Source: CAD feature listing. Evaluate the final solid. Frame: model axes, mm. A direction names the side the tool comes from. Give positions to 0.01 mm unless a question says otherwise; leave off trailing zeros. Loops run counter-clockwise (first coordinate to the right, second up) from the corner with the lowest first, then second, coordinate; pieces in that order, holes last. Notation, with made-up numbers: (3.5, 11.25) -> (44.5, 11.25) arc R26 ccw to (44.5, 35.25) -> close; hole circle Ø8 at (-8.75, 76). An arc over 180 degrees is marked (long way). Put each result on its own line as item: value.
```python
from build123d import *

# Parameters (mm, degrees)
SALIENTE_EXTRUIR2_DEPTH    = 25
CROQUIS4_W                 = 40
CROQUIS4_H                 = 40
CORTAR_EXTRUIR1_DEPTH      = 20
CROQUIS5_R                 = 7
CORTAR_EXTRUIR2_DEPTH      = 42
CORTAR_EXTRUIR2_DEPTH_BACK = 2
CROQUIS6_R                 = 4.5
CORTAR_EXTRUIR3_DEPTH      = 51
CORTAR_EXTRUIR3_DEPTH_BACK = 11
CORTAR_EXTRUIR4_DEPTH      = 26
CROQUIS9_R                 = 1.5
CROQUIS9_R_2               = 3
CORTAR_EXTRUIR6_DEPTH      = 61
CROQUIS10_R                = 1.5
CROQUIS10_R_2              = 3
CORTAR_EXTRUIR7_DEPTH      = 52
CORTAR_EXTRUIR7_DEPTH_BACK = 2
CROQUIS11_W                = 17.982621029
CROQUIS11_H                = 22.653478674
CORTAR_EXTRUIR8_DEPTH      = 52
CORTAR_EXTRUIR8_DEPTH_BACK = 2
CROQUIS13_R                = 1
CORTAR_EXTRUIR9_DEPTH      = 70
CROQUIS14_R                = 1
CORTAR_EXTRUIR10_DEPTH     = 70
CROQUIS15_R                = 2
CORTAR_EXTRUIR11_DEPTH     = 1.5
CROQUIS16_R                = 2
CORTAR_EXTRUIR12_DEPTH     = 1.5
CROQUIS18_W                = 2.75
CROQUIS18_H                = 7
CORTAR_EXTRUIR13_DEPTH     = 14


with BuildPart() as part:
    # Croquis3 → Saliente-Extruir2 (new body)
    with BuildSketch(Plane.XY):
        Polygon((-5, 45), (91.5, 50), (120, 50), (120, 45), (91.5, 45), (91.5, -5), (120, -5), (120, -10), (91.5, -10), (-5, -5), align=None)
    extrude(amount=SALIENTE_EXTRUIR2_DEPTH)

    # Croquis4 → Cortar-Extruir1 (cut)
    with BuildSketch(Plane.XY.offset(25)):
        with Locations((20, 20)):
            Rectangle(CROQUIS4_W, CROQUIS4_H)
    extrude(amount=-CORTAR_EXTRUIR1_DEPTH, mode=Mode.SUBTRACT)

    # Croquis5 → Cortar-Extruir2 (cut, two sides)
    with BuildSketch(Plane.XZ.offset(-40)) as cortar_extruir2_sk:
        with BuildLine():
            ThreePointArc((3, 15), (10, 22), (17, 15))
            Line((17, 15), (17, 25))
            Line((17, 25), (3, 25))
            Line((3, 25), (3, 15))
        make_face()
        with Locations((10, 15)):
            Circle(CROQUIS5_R)
    extrude(amount=CORTAR_EXTRUIR2_DEPTH, mode=Mode.SUBTRACT)
    extrude(cortar_extruir2_sk.sketch, amount=-CORTAR_EXTRUIR2_DEPTH_BACK, mode=Mode.SUBTRACT)

    # Croquis6 → Cortar-Extruir3 (cut, two sides)
    with BuildSketch(Plane.XZ.offset(-40)) as cortar_extruir3_sk:
        with Locations((10, 15)):
            Circle(CROQUIS6_R)
        with BuildLine():
            ThreePointArc((5.5, 15), (10, 19.5), (14.5, 15))
            Line((14.5, 15), (14.5, 25))
            Line((14.5, 25), (5.5, 25))
            Line((5.5, 25), (5.5, 15))
        make_face()
    extrude(amount=CORTAR_EXTRUIR3_DEPTH, mode=Mode.SUBTRACT)
    extrude(cortar_extruir3_sk.sketch, amount=-CORTAR_EXTRUIR3_DEPTH_BACK, mode=Mode.SUBTRACT)

    # Croquis7 → Cortar-Extruir4 (cut, through all)
    with BuildSketch(Plane.XY.offset(25)):
        Polygon((91.5, -5), (50, -0.970873786), (50, 40.970873786), (91.5, 45), align=None)
        Polygon((14.5, 45), (40, 45), (40, 47.331606218), (14.5, 46.010362694), align=None)
        Polygon((14.5, 46.010362694), (40, 47.331606218), (0.618282838, 66.022921742), (-9.359597555, 45), (-5, 45), (14.5, 45), align=None)
        Polygon((40, -7.331606218), (40, -5), (14.5, -5), (14.5, -6.010362694), align=None)
        Polygon((40, -13.475953965), (40, -7.331606218), (14.5, -6.010362694), (14.5, -5), (-5, -5), (-6.220267397, -9.241340311), align=None)
    extrude(amount=-CORTAR_EXTRUIR4_DEPTH, mode=Mode.SUBTRACT)

    # Croquis9 → Cortar-Extruir6 (cut)
    with BuildSketch(Plane(origin=(0, 50, 0), x_dir=(1, 0, 0), z_dir=(0, 1, 0))):
        with Locations((110, -8)):
            Circle(CROQUIS9_R)
        with Locations((110, -15)):
            Circle(CROQUIS9_R_2)
        with Locations((117, -15)):
            Circle(CROQUIS9_R)
        with Locations((110, -22)):
            Circle(CROQUIS9_R)
        with Locations((103, -15)):
            Circle(CROQUIS9_R)
    extrude(amount=-CORTAR_EXTRUIR6_DEPTH, mode=Mode.SUBTRACT)

    # Croquis10 → Cortar-Extruir7 (cut, two sides)
    with BuildSketch(Plane.XZ.offset(-45)) as cortar_extruir7_sk:
        with BuildLine():
            ThreePointArc((120, 18.201562119), (117.424621202, 22.424621202), (113.201562119, 25))
            Line((113.201562119, 25), (106.798437881, 25))
            ThreePointArc((106.798437881, 25), (99.625753039, 13.379814825), (110, 4.5))
            ThreePointArc((110, 4.5), (116.190056452, 6.518655701), (120, 11.798437881))
            Line((120, 11.798437881), (120, 18.201562119))
        make_face()
        with Locations((110, 8)):
            Circle(CROQUIS10_R, mode=Mode.SUBTRACT)
        with Locations((117, 15)):
            Circle(CROQUIS10_R, mode=Mode.SUBTRACT)
        with Locations((103, 15)):
            Circle(CROQUIS10_R, mode=Mode.SUBTRACT)
        with Locations((110, 15)):
            Circle(CROQUIS10_R_2, mode=Mode.SUBTRACT)
        with Locations((110, 22)):
            Circle(CROQUIS10_R, mode=Mode.SUBTRACT)
        with BuildLine():
            Line((132.305371991, 25.5), (110, 25.5))
            ThreePointArc((110, 25.5), (111.620185175, 25.374246961), (113.201562119, 25))
            Line((113.201562119, 25), (120, 25))
            Line((120, 25), (120, 18.201562119))
            ThreePointArc((120, 18.201562119), (120.374246961, 16.620185175), (120.5, 15))
            ThreePointArc((120.5, 15), (120.374246961, 13.379814825), (120, 11.798437881))
            Line((120, 11.798437881), (120, 4.5))
            Line((120, 4.5), (132.305371991, 4.5))
            Line((132.305371991, 4.5), (132.305371991, 25.5))
        make_face()
    extrude(amount=CORTAR_EXTRUIR7_DEPTH, mode=Mode.SUBTRACT)
    extrude(cortar_extruir7_sk.sketch, amount=-CORTAR_EXTRUIR7_DEPTH_BACK, mode=Mode.SUBTRACT)

    # Croquis11 → Cortar-Extruir8 (cut, two sides)
    with BuildSketch(Plane(origin=(0, -5, 0), x_dir=(1, 0, 0), z_dir=(0, 1, 0))) as cortar_extruir8_sk:
        with Locations((118.991310515, -15.826739337)):
            Rectangle(CROQUIS11_W, CROQUIS11_H)
    extrude(amount=CORTAR_EXTRUIR8_DEPTH, mode=Mode.SUBTRACT)
    extrude(cortar_extruir8_sk.sketch, amount=-CORTAR_EXTRUIR8_DEPTH_BACK, mode=Mode.SUBTRACT)

    # Croquis13 → Cortar-Extruir9 (cut)
    with BuildSketch(Plane(origin=(0, 0, 0), x_dir=(1, 0, 0), z_dir=(0, 1, 0))):
        with Locations((37.5, -7.5)):
            Circle(CROQUIS13_R)
        with Locations((37.5, -22.5)):
            Circle(CROQUIS13_R)
        with Locations((22.5, -22.5)):
            Circle(CROQUIS13_R)
        with Locations((22.5, -7.5)):
            Circle(CROQUIS13_R)
    extrude(amount=CORTAR_EXTRUIR9_DEPTH, mode=Mode.SUBTRACT)

    # Croquis14 → Cortar-Extruir10 (cut)
    with BuildSketch(Plane(origin=(0, 0, 0), x_dir=(1, 0, 0), z_dir=(0, 1, 0))):
        with Locations((37.071067812, -15)):
            Circle(CROQUIS14_R)
        with Locations((30, -7.928932188)):
            Circle(CROQUIS14_R)
        with Locations((30, -22.071067812)):
            Circle(CROQUIS14_R)
    extrude(amount=-CORTAR_EXTRUIR10_DEPTH, mode=Mode.SUBTRACT)

    # Croquis15 → Cortar-Extruir11 (cut)
    with BuildSketch(Plane(origin=(0, 45, 0), x_dir=(1, 0, 0), z_dir=(0, 1, 0))):
        with Locations((22.5, -7.5)):
            Circle(CROQUIS15_R)
        with Locations((37.5, -7.5)):
            Circle(CROQUIS15_R)
        with Locations((37.5, -22.5)):
            Circle(CROQUIS15_R)
        with Locations((22.5, -22.5)):
            Circle(CROQUIS15_R)
    extrude(amount=-CORTAR_EXTRUIR11_DEPTH, mode=Mode.SUBTRACT)

    # Croquis16 → Cortar-Extruir12 (cut)
    with BuildSketch(Plane.XZ.offset(5)):
        with Locations((30, 22.071067812)):
            Circle(CROQUIS16_R)
        with Locations((37.071067812, 15)):
            Circle(CROQUIS16_R)
        with Locations((30, 7.928932188)):
            Circle(CROQUIS16_R)
    extrude(amount=-CORTAR_EXTRUIR12_DEPTH, mode=Mode.SUBTRACT)

    # Croquis18 → Cortar-Extruir13 (cut)
    with BuildSketch(Plane.XY.offset(25)):
        with Locations((-1.375, 29.5)):
            Rectangle(CROQUIS18_W, CROQUIS18_H)
    extrude(amount=-CORTAR_EXTRUIR13_DEPTH, mode=Mode.SUBTRACT)


solid = part.part
```
(1) Section D-D on x = 84. Return loops of the section in (y, z).
Calculated:
outline: (-9.61, 0) -> (-4.27, 0) -> (-4.27, 25) -> (-9.61, 25) -> close; (44.27, 0) -> (49.61, 0) -> (49.61, 25) -> (44.27, 25) -> close
(2) First-contact query: P1, Ø2.5, axis at x = 37.5, z = 22.5, coming from the +Y side; P2, Ø1.5, axis at y = 21.5, z = 12, coming from the +X side; P3, Ø2, axis at x = -1, z = 19.5, coming from the +Y side. Flat tips, straight axial feed; report the tip coordinate or a pass-through.
Calculated:
P1: stops at y = 43.5
P2: stops at x = 50
P3: stops at y = 45
(3) Section B-B on x = 59.5. Return loops of the section in (y, z).
Calculated:
outline: (-8.34, 0) -> (-1.89, 0) -> (-1.89, 25) -> (-8.34, 25) -> close; (41.89, 0) -> (48.34, 0) -> (48.34, 25) -> (41.89, 25) -> close
(4) Reachability of faces 4 (the flat face through (40, 20, 15)), 5 (the flat face through (112, -7, 12)), 6 (the cylindrical face through (31.908, -4.26, 8.53)), 7 (the flat face through (17, 45, 13)) from +Z, -Z, +X, -X, +Y, -Y: full face, straight path, thin tool, end or side. Return the list, or none.
Calculated:
face 4: +Z
face 5: +X
face 6: -Y
face 7: +Z, -Z, -X, +Y
(5) Section A-A on y = 2.5. Return loops of the section in (x, z), then the cut area to 3 significant figures.
Calculated:
outline: (-5, 0) -> (50, 0) -> (50, 25) -> (40, 25) -> (40, 5) -> (0, 5) -> (0, 25) -> (-5, 25) -> close
area: 575 mm²
(6) Line query: probe 1 along Z at (x, y) = (22.5, 42.4); probe 2 along Z at (x, y) = (110, 48); probe 3 along X at (y, z) = (1.5, 11). Output: solid intervals per line, ascending. Write a range as from..to.
Calculated:
probe 1: z = 0..6.5, 8.5..21.5, 23.5..25
probe 2: z = 0..6.5, 9.5..12, 18..20.5, 23.5..25
probe 3: x = -5..0, 40..50
(7) Draft query along X for faces 1 (the flat face through (40, 46, 13)), 2 (the flat face through (99, -5, 10)), 3 (the cylindrical face through (9.9, 43.5, 10.5)). Return one class per face: released by +X, released by -X, zero draft, split by the parting line, or undercut.
Calculated:
face 1: released by -X
face 2: zero draft
face 3: undercut
(8) Section C-C on x = 10. Return loops of the section in (y, z), then the cut area to 3 significant figures.
Calculated:
outline: (-5, 0) -> (45, 0) -> (45, 10.5) -> (42, 10.5) -> (42, 8) -> (40, 8) -> (40, 5) -> (0, 5) -> (0, 8) -> (-2, 8) -> (-2, 10.5) -> (-5, 10.5) -> close
area: 295 mm²
